Can you work these out from the model? Positions are in its coordinate system, mm. A direction names the side the tool comes from. Coordinates: 2 decimals unless noted, no trailing zeros. Order: outer loops, then holes, each group sorted by start corner. A loop starts at its lowest first (then second) coordinate and runs counter-clockwise, first axis right, second up.
```python
from build123d import *

# Parameters (mm, degrees)
F0_W     = 31.6056316875
F0_H     = 12
F1_DEPTH = 25
F2_W     = 8.3738705143
F2_H     = 14.6988127381
F3_DEPTH = 166
F4_W     = 7.847521259
F4_H     = 27.2596180439
F5_DEPTH = 5


# Not quite as in the source:
# - an extrude ends at something that could not be found from the text; its depth is read off the source's solid


with BuildPart() as f1:
    # F0 (on Top) → F1 (new body)
    with BuildSketch(Plane.XY):
        Polygon((48.9295756356, -27.3802791548), (48.9295756356, 27.3802791548), (-48.9295756356, 27.3802791548), (-48.9295756356, 6), (-17.3239439482, 6), (-17.3239439482, -6), (-48.9295756356, -6), (-48.9295756356, -27.3802791548), align=None)
        with Locations((-33.1267597919, 0)):
            Rectangle(F0_W, F0_H)
    extrude(amount=F1_DEPTH)

    # F2 (on face) → F3 (cut, through all)
    with BuildSketch(Plane.YZ.offset(48.9295756356)):
        with Locations((0, -7.349406369)):
            Rectangle(F2_W, F2_H)
        Polygon((13.6298090219, 11.6699673235), (13.6298090219, 18.7966637313), (-13.6298090219, 18.7966637313), (-13.6298090219, 11.6699673235), (-4.1869352572, 11.6699673235), (-4.1869352572, 0), (4.1869352572, 0), (4.1869352572, 11.6699673235), align=None)
    extrude(amount=-F3_DEPTH, mode=Mode.SUBTRACT)

    # F4 (on face) → F5 (join)
    with BuildSketch(Plane(origin=(0, 0, 18.7966637313), x_dir=(1, 0, 0), z_dir=(0, 0, -1))):
        with Locations((-45.0058150061, 0)):
            Rectangle(F4_W, F4_H)
        with Locations((45.0058150061, 0)):
            Rectangle(F4_W, F4_H)
    extrude(amount=F5_DEPTH)


solid = f1.part
```
1. Imagine slicing it at B-B on z = 7.25. Please give me the cut outline in (x, y), then the cut area to 3 significant figures.
Completed:
outline: (-48.93, -27.38) - (48.93, -27.38) - (48.93, -4.19) - (-48.93, -4.19) - close; (-48.93, 4.19) - (48.93, 4.19) - (48.93, 27.38) - (-48.93, 27.38) - close
area: 4,540 mm2
2. I'm going to push a flat-ended pin straight in: pin 1 (6 mm diameter, centred on y = -0.5, z = 5, fed in from -X). Where does the tip first touch, or does it pass through?
Completed:
pin 1: passes through
3. Imagine slicing it at A-A on y = -9. Please give me the cut outline in (x, z), then the cut area to 3 significant figures.
Completed:
outline: (-48.93, 0) - (48.93, 0) - (48.93, 11.67) - (-48.93, 11.67) - close; (-48.93, 13.8) - (-41.08, 13.8) - (-41.08, 18.8) - (41.08, 18.8) - (41.08, 13.8) - (48.93, 13.8) - (48.93, 25) - (-48.93, 25) - close
area: 1,830 mm2
4. Imagine slicing it at C-C on x = -14.5. Please give me the cut outline in (y, z).
Completed:
outline: (-27.38, 0) - (-4.19, 0) - (-4.19, 11.67) - (-13.63, 11.67) - (-13.63, 18.8) - (13.63, 18.8) - (13.63, 11.67) - (4.19, 11.67) - (4.19, 0) - (27.38, 0) - (27.38, 25) - (-27.38, 25) - close
5. On a 3-axis mill with a long thin cutter (end or side, diameter ignored), from which of +Z, -Z, +X, -X, +Y, -Y can I reach the whole of each face in a straight line? I mean faces 4 (the flat face through (-45, 0, 13.797)), 5 (the flat face through (1, -4.187, 6)), 6 (the flat face through (1, -13.63, 15)). Say none if no direction works.
Completed:
face 4: +X, -X
face 5: -Z, +X, -X
face 6: none
6. Please list where these lines run through material, in increasing order: probe 1 along Y at (x, z) = (27.5, 12.5); probe 2 along Y at (x, z) = (-41.5, 2.5); probe 3 along Z at (x, y) = (30.5, 7).
Completed:
probe 1: y = -27.38 to -13.63, 13.63 to 27.38
probe 2: y = -27.38 to -4.19, 4.19 to 27.38
probe 3: z = 0 to 11.67, 18.8 to 25
7. Thinking about a two-plate mould opening in Y: for faces 1 (the flat face through (1, 9, 11.67)), 2 (the flat face through (-48.93, 0, 15)), 3 (the flat face through (-1, -27.38, 12)), which applies, pulls with the +Y half, pulls with the -Y half, needs draft (parallel to the pull), parting line crosses it, or undercut?
Completed:
face 1: undercut
face 2: needs draft
face 3: pulls with the -Y half
8. Imagine slicing it at D-D on y = 1.5. Please give me the cut outline in (x, z), then the cut area to 3 significant figures.
Completed:
outline: (-48.93, 13.8) - (-41.08, 13.8) - (-41.08, 18.8) - (41.08, 18.8) - (41.08, 13.8) - (48.93, 13.8) - (48.93, 25) - (-48.93, 25) - close
area: 686 mm2
